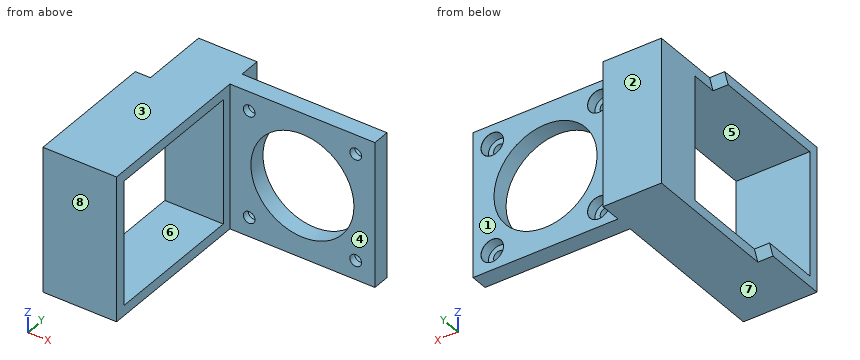
```python
from build123d import *

# Parameters (mm, degrees)
SKETCH1_W                     = 42.2
SKETCH1_H                     = 58.25
BOSS_EXTRUDE1_DEPTH           = 17
SKETCH2_W                     = 42.2
SKETCH2_H                     = 5
BOSS_EXTRUDE2_DEPTH           = 42.2
CBORE_FOR_M3_SHCS1_AT_2_COUNT = 2
CBORE_FOR_M3_SHCS1_AT_2_PITCH = 31
CBORE_FOR_M3_SHCS1_AT_3_COUNT = 2
CBORE_FOR_M3_SHCS1_AT_3_PITCH = 43.840620434
CBORE_FOR_M3_SHCS1_AT_4_COUNT = 2
CBORE_FOR_M3_SHCS1_AT_4_PITCH = 31
SKETCH5_R                     = 15
CUT_EXTRUDE1_DEPTH            = 53
BOSS_EXTRUDE3_DEPTH           = 4.4
SKETCH7_W                     = 36.2
SKETCH7_H                     = 41.25
CUT_EXTRUDE2_DEPTH            = 22.4


with BuildPart() as part:
    # Sketch1 → Boss-Extrude1 (new body)
    with BuildSketch(Plane(origin=(0, 0, 0), x_dir=(0, 0, -1), z_dir=(1, 0, 0))):
        with Locations((0, 29.125)):
            Rectangle(SKETCH1_W, SKETCH1_H)
    extrude(amount=BOSS_EXTRUDE1_DEPTH)

    # Sketch2 → Boss-Extrude2 (add)
    with BuildSketch(Plane(origin=(17, 0, 0), x_dir=(0, 0, -1), z_dir=(1, 0, 0))):
        with Locations((0, 49.5)):
            Rectangle(SKETCH2_W, SKETCH2_H)
    extrude(amount=BOSS_EXTRUDE2_DEPTH)

    # Sketch4 → CBORE for M3 SHCS1 (revolve, cut)
    with BuildSketch(Plane(origin=(53.6, 52, 15.5), x_dir=(0, 0, 1), z_dir=(1, 0, 0))):
        Polygon((0, 0), (0, 52), (1.7, 52), (1.7, 3), (3.25, 3), (3.25, 0.025), (3.275, 0), align=None)
    cbore_for_m3_shcs1 = revolve(axis=Axis((53.6, 58.35, 15.5), (0, -1, 0)), mode=Mode.SUBTRACT)

    # CBORE for M3 SHCS1 at 2: CBORE for M3 SHCS1 ×2
    with Locations(*[(0, 0, -i * CBORE_FOR_M3_SHCS1_AT_2_PITCH) for i in range(1, CBORE_FOR_M3_SHCS1_AT_2_COUNT)]):
        add(cbore_for_m3_shcs1, mode=Mode.SUBTRACT)

    # CBORE for M3 SHCS1 at 3: CBORE for M3 SHCS1 ×2
    with Locations(*[Vector(-0.707106781, 0, -0.707106781) * (i * CBORE_FOR_M3_SHCS1_AT_3_PITCH) for i in range(1, CBORE_FOR_M3_SHCS1_AT_3_COUNT)]):
        add(cbore_for_m3_shcs1, mode=Mode.SUBTRACT)

    # CBORE for M3 SHCS1 at 4: CBORE for M3 SHCS1 ×2
    with Locations(*[(-i * CBORE_FOR_M3_SHCS1_AT_4_PITCH, 0, 0) for i in range(1, CBORE_FOR_M3_SHCS1_AT_4_COUNT)]):
        add(cbore_for_m3_shcs1, mode=Mode.SUBTRACT)

    # Sketch5 → Cut-Extrude1 (cut, through all)
    with BuildSketch(Plane(origin=(0, 52, 0), x_dir=(1, 0, 0), z_dir=(0, 1, 0))):
        with Locations((38.1, 0)):
            Circle(SKETCH5_R)
    extrude(amount=-CUT_EXTRUDE1_DEPTH, mode=Mode.SUBTRACT)

    # Sketch6 → Boss-Extrude3 (add)
    with BuildSketch(Plane(origin=(0, 0, 0), x_dir=(0, 0, -1), z_dir=(1, 0, 0))):
        Polygon((-21.1, 38.25), (21.1, 18.25), (21.1, 0), (-21.1, 0), align=None)
    extrude(amount=-BOSS_EXTRUDE3_DEPTH)

    # Sketch7 → Cut-Extrude2 (cut, through all)
    with BuildSketch(Plane(origin=(17, 0, 0), x_dir=(0, 0, -1), z_dir=(1, 0, 0))):
        with Locations((0, 23.625)):
            Rectangle(SKETCH7_W, SKETCH7_H)
    extrude(amount=-CUT_EXTRUDE2_DEPTH, mode=Mode.SUBTRACT)


solid = part.part
```
Read the model definition and answer for the solid it produces. Units are mm, in the model's axes. Face numbers are marked on the shaded views. A direction names the side the tool comes from. Coordinates: 2 decimals unless noted, no trailing zeros. Write each loop counter-clockwise with the first axis right and the second up, starting at its lowest first coordinate (ties: lowest second). Pieces come first, ordered by that corner, then holes. Notation, with made-up numbers: (-13, -12.75) - (41, -12.75) arc R26 ccw to (41, 15.25) - close; hole circle Ø5 at (-30.5, 72). An arc over 180 degrees is marked (long way). Answer as a JSON object with one key per item and string values. Group by question number.
1. A cutting plane is placed at D-D (x = 38.1). Determine the outline of the cut face in (y, z), plus the area to 3 significant figures.
2. Each of these flat-tipped pins is pushed along its axis until it touches: P1, Ø2, axis at x = 22.5, z = -14.5, coming from the +Y side; P2, Ø12, axis at x = 24, y = 14.5, coming from the -Z side; P3, Ø3, axis at y = 55, z = -4.5, coming from the +X side; P4, Ø8.5, axis at x = 53.6, z = 15.5, coming from the -Y side. Where does it stop, or does it pass through?
3. A cutting plane is placed at C-C (z = 0). Determine the outline of the cut face in (x, y).
4. The mould has two halves that part along Z. Classify the marked faces 6, 7 and 8: +Z half, -Z half, draft (parallel to the pull), parting line (faces both ways), or undercut.
5. A cutting plane is placed at B-B (y = 11.5). Determine the outline of the cut face in (x, z), plus the area to 3 significant figures.
6. Which of the six approach directions +Z, -Z, +X, -X, +Y, -Y give full straight-line access (tool end or side, diameter ignored) to the marked faces 1, 2, 3, 4 and 5?
7. Consider L1, parallel to Z at x = 53.6, y = 48.3; L2, parallel to X at y = 48.4, z = 15.5; L3, parallel to Z at x = 53.6, y = 50.3. Determine where each line is inside the solid, lowest interval first. Write a range as [from, to].
8. A cutting plane is placed at A-A (x = 15). Determine the outline of the cut face in (y, z).
Worked out:
{
 "1": {"outline": "(47, -21.1) - (52, -21.1) - (52, -15) - (47, -15) - close; (47, 15) - (52, 15) - (52, 21.1) - (47, 21.1) - close", "area": "61.0 mm²"},
 "2": {"P1": "stops at y = 49", "P2": "passes through", "P3": "stops at x = 17", "P4": "stops at y = 47"},
 "3": {"outline": "(-4.4, 0) - (17, 0) - (17, 3) - (-4.4, 3) - close; (0, 44.25) - (17, 44.25) - (17, 47) - (23.1, 47) - (23.1, 52) - (17, 52) - (17, 58.25) - (0, 58.25) - close; (53.1, 47) - (59.2, 47) - (59.2, 52) - (53.1, 52) - close"},
 "4": {"face 6": "undercut", "face 7": "-Z half", "face 8": "draft"},
 "5": {"outline": "(-4.4, -21.1) - (17, -21.1) - (17, -18.1) - (-4.4, -18.1) - close; (-4.4, 18.1) - (17, 18.1) - (17, 21.1) - (-4.4, 21.1) - close", "area": "128 mm²"},
 "6": {"face 1": "+Z, -Z, +X, +Y", "face 2": "+Z, -Z, +X, -X, +Y", "face 3": "+Z, +X, -X, +Y, -Y", "face 4": "+Z, -Z, +X, -Y", "face 5": "+X, -X"},
 "7": {"L1": "z = [-21.1, -17.2], [-13.8, 13.8], [17.2, 21.1]", "L2": "x = [0, 20.9], [24.3, 51.9], [55.3, 59.2]", "L3": "z = [-21.1, -18.75], [-12.25, 12.25], [18.75, 21.1]"},
 "8": {"outline": "(0, -21.1) - (58.25, -21.1) - (58.25, 21.1) - (0, 21.1) - close; hole (3, -18.1) - (44.25, -18.1) - (44.25, 18.1) - (3, 18.1) - close"}
}
